Autodesk Inventor part; units mm, degrees
ref_plane "YZ Plane" through (0, 0, 0) normal (1, 0, 0) x (0, 1, 0)
ref_plane "XZ Plane" through (0, 0, 0) normal (0, 1, 0) x (-1, 0, 0)
ref_plane "XY Plane" through (0, 0, 0) normal (0, 0, 1) x (1, 0, 0)
sketch "Sketch3" plane through (0, 0, 0) normal (0, 0, 1) x (1, 0, 0)
  line L0 (0, 0) -> (0, 7)
  line L1 (0, 7) -> (-20, 7)
  line L2 (-20, 7) -> (-20, 0)
  line L3 (-20, 0) -> (-15, 0)
  line L4 (-15, 0) -> (-15, 5)
  line L5 (-15, 5) -> (-5, 5)
  line L6 (-15, 5) -> (-5, 5) construction
  line L7 (-5, 5) -> (-5, 0)
  line L8 (-5, 0) -> (0, 0)
  dimension "d22" = 7
  dimension "d23" = 20
  dimension "d24" = 90
  dimension "d25" = 7
  dimension "d26" = 90
  dimension "d27" = 5
  dimension "d28" = 90
  dimension "d29" = 5
  dimension "d30" = 10
  dimension "d31" = 0
  dimension "d32" = 5
  dimension "d33" = 90
extrude "Extrusion3" add sketch "Sketch3" along normal blind 150
fillet "Fillet4" radius 1 20 edges at (-15, 2.5, 150) (-10, 5, 150) (-5, 2.5, 150) (-5, 2.5, 0) (-5, 0, 75) (-2.5, 0, 150) (0, 3.5, 150) (0, 0, 75) (0, 3.5, 0) (-10, 7, 150) (-20, 3.5, 150) (-17.5, 0, 150) (-15, 0, 75) (-15, 2.5, 0) (-20, 3.5, 0) (-20, 0, 75) (-10, 7, 0) (-10, 5, 0) (-2.5, 0, 0) (-17.5, 0, 0)
fillet "Fillet5" radius 1 2 edges at (-4.7071, 5.2929, 149.7071) (-15.2929, 5.2929, 149.7071)
fillet "Fillet6" radius 1 6 edges at (-0.2929, 6.7071, 149.7071) (-0.2929, 6.7071, 0.2929) (0, 7, 75) (-19.7071, 6.7071, 149.7071) (-19.7071, 6.7071, 0.2929) (-20, 7, 75)
properties part number "Cable_Cover"
Can you work these out from the model? Positions are in its coordinate system, mm. A direction names the side the tool comes from. Coordinates: 2 decimals unless noted, no trailing zeros. Order: outer loops, then holes, each group sorted by start corner. A loop starts at its lowest first (then second) coordinate and runs counter-clockwise, first axis right, second up.
1. I need wall thicknesses on line 1 (X direction, y = 3, z = 78); line 2 (Y direction, x = -10.75, z = 6); line 3 (X direction, y = 4.5, z = 138). Which ranges of each line are inside material? Lowest first, please.
2. If we section it at A-A (z = 122): Please give me the cut outline in (x, y), then the cut area to 3 significant figures.
3. Thinking about a two-plate mould opening in X: for faces 3 (the face through (-3, 0, 74)), 4 (the face through (-20, 4, 74)), 5 (the face through (-5, 3, 74)), which applies, +X half, -X half, draft (parallel to the pull), parting line (faces both ways), or undercut?
4. I'm going to push a flat-ended pin straight in: pin 1 (2 mm diameter, centred on x = -11, z = 102.5, fed in from -Y). Where does the tip first touch, or does it pass through?
5. For faces 1 (the face through (-10, 5, 74)), 2 (the face through (-10, 7, 74)), which set-ups out of +Z, -Z, +X, -X, +Y, -Y let a thin tool reach every point of the face, with its end or its side?
Entries:
1. line 1: x = -20 to -15, -5 to 0
1. line 2: y = 5 to 7
1. line 3: x = -20 to -14.87, -5.13 to 0
2. outline: (-20, 1) arc R1 ccw to (-19, 0) - (-16, 0) arc R1 ccw to (-15, 1) - (-15, 4) arc R1 cw to (-14, 5) - (-6, 5) arc R1 cw to (-5, 4) - (-5, 1) arc R1 ccw to (-4, 0) - (-1, 0) arc R1 ccw to (0, 1) - (0, 6) arc R1 ccw to (-1, 7) - (-19, 7) arc R1 ccw to (-20, 6) - close
2. area: 89.1 mm2
3. face 3: draft
3. face 4: -X half
3. face 5: undercut
4. pin 1: stops at y = 5
5. face 1: +Z, -Z, -Y
5. face 2: +Z, -Z, +X, -X, +Y
